Design review of the part built by this model. Coordinates are the model's own, in mm. Give positions to 0.01 mm unless a question says otherwise; leave off trailing zeros. Order: outer loops, then holes, each group sorted by start corner. A loop starts at its lowest first (then second) coordinate and runs counter-clockwise, first axis right, second up. Notation, with made-up numbers: (81.5, 3) - (103.5, 3) arc R26 ccw to (103.5, 35) - close; hole circle Ø6 at (-6.75, 77.25). An arc over 180 degrees is marked (long way). Write each question's results on one line, items separated by ' | '. Start each with the question number.
```python
from build123d import *

# Parameters (mm, degrees)
SKETCH1_R           = 2.552698787
SKETCH1_R_2         = 2.5527
SKETCH1_R_3         = 3.175
BOSS_EXTRUDE2_DEPTH = 3.175


with BuildPart() as part:
    # Sketch1 → Boss-Extrude2 (new, symmetric)
    with BuildSketch(Plane(origin=(0, 0, 0), x_dir=(1, 0, 0), z_dir=(0, 1, 0))):
        with BuildLine():
            Line((-28.575, -15.875), (28.575, -15.875))
            add(Edge.make_bspline(
                [(28.575, -15.875), (29.157862345, -15.875), (29.730465383, -15.768989089), (30.338469644, -15.656424047), (30.912401406, -15.429155712), (31.511428211, -15.191950117), (32.049781934, -14.839921496), (32.600578196, -14.479756719), (33.065128061, -14.015128061), (33.530435301, -13.549741898), (33.889921496, -12.999781934), (34.242433686, -12.460491153), (34.479155712, -11.862401406), (34.706715402, -11.287460745), (34.818989089, -10.680465383), (34.925, -10.107329034), (34.925, -9.525)],
                knots=[0, 0, 0, 0.125, 0.125, 0.25, 0.25, 0.375, 0.375, 0.5, 0.5, 0.625, 0.625, 0.75, 0.75, 0.875, 0.875, 1, 1, 1], degree=2))
            Line((34.925, -9.525), (34.925, 9.525))
            add(Edge.make_bspline(
                [(34.925, 9.525), (34.925, 10.107862345), (34.818989089, 10.680465383), (34.706424047, 11.288469644), (34.479155712, 11.862401406), (34.241950117, 12.461428211), (33.889921496, 12.999781934), (33.529756719, 13.550578196), (33.065128061, 14.015128061), (32.599741898, 14.480435301), (32.049781934, 14.839921496), (31.510491153, 15.192433686), (30.912401406, 15.429155712), (30.337460745, 15.656715402), (29.730465383, 15.768989089), (29.157329034, 15.875), (28.575, 15.875)],
                knots=[0, 0, 0, 0.125, 0.125, 0.25, 0.25, 0.375, 0.375, 0.5, 0.5, 0.625, 0.625, 0.75, 0.75, 0.875, 0.875, 1, 1, 1], degree=2))
            Line((28.575, 15.875), (-28.575, 15.875))
            add(Edge.make_bspline(
                [(-28.575, 15.875), (-29.157862345, 15.875), (-29.730465383, 15.768989089), (-30.338469644, 15.656424047), (-30.912401406, 15.429155712), (-31.511428211, 15.191950117), (-32.049781934, 14.839921496), (-32.600578196, 14.479756719), (-33.065128061, 14.015128061), (-33.530435301, 13.549741898), (-33.889921496, 12.999781934), (-34.242433686, 12.460491153), (-34.479155712, 11.862401406), (-34.706715402, 11.287460745), (-34.818989089, 10.680465383), (-34.925, 10.107329034), (-34.925, 9.525)],
                knots=[0, 0, 0, 0.125, 0.125, 0.25, 0.25, 0.375, 0.375, 0.5, 0.5, 0.625, 0.625, 0.75, 0.75, 0.875, 0.875, 1, 1, 1], degree=2))
            Line((-34.925, 9.525), (-34.925, -9.525))
            add(Edge.make_bspline(
                [(-34.925, -9.525), (-34.925, -10.107862345), (-34.818989089, -10.680465383), (-34.706424047, -11.288469644), (-34.479155712, -11.862401406), (-34.241950117, -12.461428211), (-33.889921496, -12.999781934), (-33.529756719, -13.550578196), (-33.065128061, -14.015128061), (-32.599741898, -14.4804353), (-32.049781934, -14.839921496), (-31.510491153, -15.192433686), (-30.912401406, -15.429155712), (-30.337460745, -15.656715402), (-29.730465383, -15.768989089), (-29.157329034, -15.875), (-28.575, -15.875)],
                knots=[0, 0, 0, 0.125, 0.125, 0.25, 0.25, 0.375, 0.375, 0.5, 0.5, 0.625, 0.625, 0.75, 0.75, 0.875, 0.875, 1, 1, 1], degree=2))
        make_face()
        with Locations(Location((-9.525, -9.525, 0), (0, 0, 270))):
            Circle(SKETCH1_R, mode=Mode.SUBTRACT)
        with Locations(Location((-9.525, 9.525, 0), (0, 0, 270))):
            Circle(SKETCH1_R_2, mode=Mode.SUBTRACT)
        with Locations(Location((-26.67, 0, 0), (0, 0, 270))):
            Circle(SKETCH1_R_3, mode=Mode.SUBTRACT)
        with Locations(Location((0, -9.525, 0), (0, 0, 270))):
            Circle(SKETCH1_R_2, mode=Mode.SUBTRACT)
        with Locations(Location((9.525, -9.525, 0), (0, 0, 270))):
            Circle(SKETCH1_R_2, mode=Mode.SUBTRACT)
        with Locations(Location((26.67, 0, 0), (0, 0, 270))):
            Circle(SKETCH1_R_3, mode=Mode.SUBTRACT)
        with Locations(Location((9.525, 9.525, 0), (0, 0, 270))):
            Circle(SKETCH1_R_2, mode=Mode.SUBTRACT)
        with Locations(Location((0, 9.525, 0), (0, 0, 270))):
            Circle(SKETCH1_R_2, mode=Mode.SUBTRACT)
        with Locations(Location((0, 0, 0), (0, 0, 270))):
            Circle(SKETCH1_R_2, mode=Mode.SUBTRACT)
    extrude(amount=BOSS_EXTRUDE2_DEPTH, both=True)


solid = part.part
```
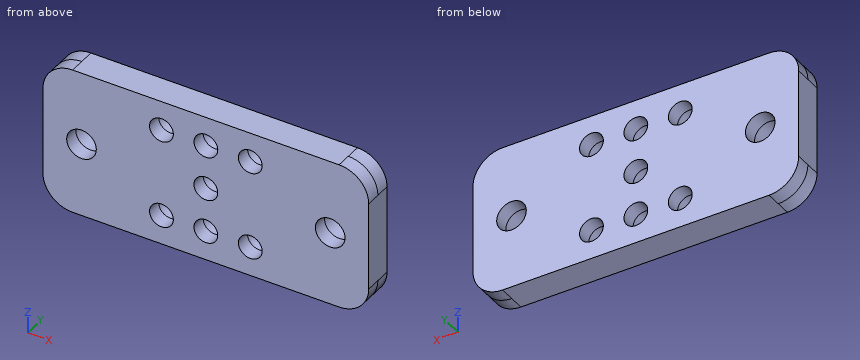
Q1. Add section D-D (y = 1.5). Give the number of separate pieces and of enclosed holes in the cut face, plus the area to 3 significant figures.
Q2. For line 1 (X direction, y = -0.5, z = -9.5) (3 decimals); line 2 (X direction, y = -0.9, z = 0) (3 decimals); line 3 (Z direction, x = -11.5, y = -1) (3 decimals), list the stretches that pass through material, from the lowest coordinate up. Write a range as [from, to].
Q3. Add section A-A (z = 0). Give the boundary of the cut face in (x, y) (3 decimals).
Q4. Add section B-B (x = 0). Give the boundary of the cut face in (y, z) (3 decimals), plus the area to 3 significant figures.
Q5. Add section C-C (x = -26.67). Give the boundary of the cut face in (y, z) (3 decimals), plus the area to 3 significant figures.
Q6. Insertion check: pin 1 Ø8 at (x, z) = (9.525, 9.525) entering from +Y (3 decimals). The pin has a flat end and moves straight along its axis. Give the tip position at first contact, or say it passes through.
Verdict:
1) separate pieces: 1 | enclosed holes: 9 | area: 1,980 mm2
2) line 1: x = [-34.925, -12.078], [-6.972, -2.553], [2.553, 6.972], [12.078, 34.925] | line 2: x = [-34.925, -29.845], [-23.495, -2.553], [2.553, 23.495], [29.845, 34.925] | line 3: z = [-15.875, -11.142], [-7.908, 7.908], [11.142, 15.875]
3) outline: (-34.925, -3.175) - (-29.845, -3.175) - (-29.845, 3.175) - (-34.925, 3.175) - close; (-23.495, -3.175) - (-2.553, -3.175) - (-2.553, 3.175) - (-23.495, 3.175) - close; (2.553, -3.175) - (23.495, -3.175) - (23.495, 3.175) - (2.553, 3.175) - close; (29.845, -3.175) - (34.925, -3.175) - (34.925, 3.175) - (29.845, 3.175) - close
4) outline: (-3.175, -15.875) - (3.175, -15.875) - (3.175, -12.078) - (-3.175, -12.078) - close; (-3.175, -6.972) - (3.175, -6.972) - (3.175, -2.553) - (-3.175, -2.553) - close; (-3.175, 2.553) - (3.175, 2.553) - (3.175, 6.972) - (-3.175, 6.972) - close; (-3.175, 12.078) - (3.175, 12.078) - (3.175, 15.875) - (-3.175, 15.875) - close | area: 104 mm2
5) outline: (-3.175, -15.875) - (3.175, -15.875) - (3.175, -3.175) - (-3.175, -3.175) - close; (-3.175, 3.175) - (3.175, 3.175) - (3.175, 15.875) - (-3.175, 15.875) - close | area: 161 mm2
6) pin 1: stops at y = 3.175
